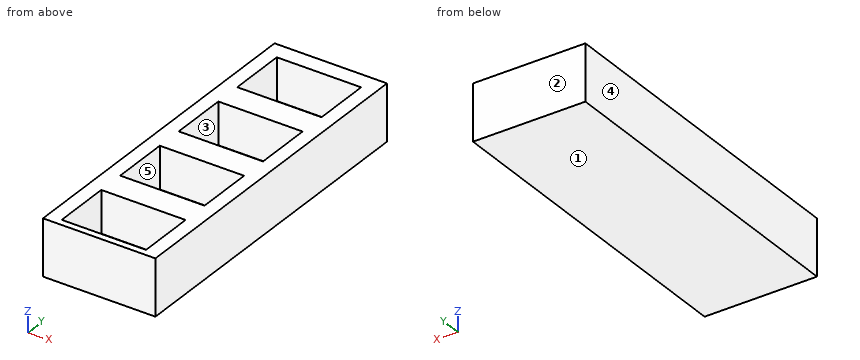
from build123d import *

# Parameters (mm, degrees)
F1_DEPTH = 25.4
F2_DEPTH = 6.35


with BuildPart() as f1:
    # F0 (on Top) → F1 (new body)
    with BuildSketch(Plane.XY):
        Polygon((25.4, -76.2), (25.4, 76.2), (0, 76.2), (-25.4, 76.2), (-25.4, -76.2), align=None)
        Polygon((-19.05, -47.105642), (0, -47.105642), (19.05, -47.105642), (19.05, -73.140642), (-19.05, -73.140642), align=None, mode=Mode.SUBTRACT)
        Polygon((-19.05, -8.599242), (0, -8.599242), (19.05, -8.599242), (19.05, -34.634242), (0, -34.634242), (-19.05, -34.634242), align=None, mode=Mode.SUBTRACT)
        Polygon((-19.05, 29.907158), (0, 29.907158), (19.05, 29.907158), (19.05, 3.872158), (0, 3.872158), (-19.05, 3.872158), align=None, mode=Mode.SUBTRACT)
        Polygon((-19.05, 68.410887), (19.05, 68.410887), (19.05, 42.375887), (0, 42.375887), (-19.05, 42.375887), align=None, mode=Mode.SUBTRACT)
    extrude(amount=F1_DEPTH)

    # F0 (on Top) → F2 (join)
    with BuildSketch(Plane.XY):
        Polygon((19.05, 42.375887), (19.05, 68.410887), (-19.05, 68.410887), (-19.05, 42.375887), (0, 42.375887), align=None)
        Polygon((19.05, 29.907158), (0, 29.907158), (0, 29.675887), (0, 16.889658), (0, 3.872158), (19.05, 3.872158), align=None)
        Polygon((0, 29.675887), (0, 29.907158), (-19.05, 29.907158), (-19.05, 3.872158), (0, 3.872158), (0, 16.889658), align=None)
        Polygon((0, -21.616742), (0, -8.599242), (-19.05, -8.599242), (-19.05, -34.634242), (0, -34.634242), align=None)
        Polygon((19.05, -8.599242), (0, -8.599242), (0, -21.616742), (0, -34.634242), (19.05, -34.634242), align=None)
        Polygon((19.05, -47.105642), (0, -47.105642), (-19.05, -47.105642), (-19.05, -73.140642), (19.05, -73.140642), align=None)
    extrude(amount=F2_DEPTH)


solid = f1.part
Verification items for the finished model (mm, model axes). Face numbers are marked on the shaded views. A direction names the side the tool comes from. Give positions to 0.01 mm unless a question says otherwise; leave off trailing zeros. Loops run counter-clockwise (first coordinate to the right, second up) from the corner with the lowest first, then second, coordinate; pieces in that order, holes last.
1) Sectioned sample at C-C, the plane y = -12. Enter the section's corners in (x, z), then the cut area to 3 significant figures.
2) Sectioned sample at B-B, the plane x = -15.5. Enter the section's corners in (y, z), then the cut area to 3 significant figures.
3) Depth check by flat-ended pin: pin 1 Ø10 at (x, y) = (4, -25.5) entering from -Z; pin 2 Ø3 at (x, y) = (9, 14.5) entering from +Z. Enter the tip coordinate at first touch or a pass-through.
4) Set-up check for the marked faces 4 and 5: record each of +Z, -Z, +X, -X, +Y, -Y from which the full face is reachable in a straight line by a thin tool's end or side.
5) Thickness scan on line 1 along Y through (x, z) = (17, 6.5); line 2 along X through (y, z) = (-26, 17); line 3 along Z through (x, y) = (-14.5, -18). Record the ranges inside material, lowest first.
6) Draft check along Y on the marked faces 1, 2 and 3. Enter one of: pulls with the +Y half, pulls with the -Y half, needs draft (parallel to the pull), parting line crosses it, or undercut.
7) Sectioned sample at A-A, the plane z = 20. Enter the section's corners in (x, y), then the cut area to 3 significant figures.
Answers:
1. outline: (-25.4, 0) - (25.4, 0) - (25.4, 25.4) - (19.05, 25.4) - (19.05, 6.35) - (-19.05, 6.35) - (-19.05, 25.4) - (-25.4, 25.4) - close
1. area: 565 mm2
2. outline: (-76.2, 0) - (76.2, 0) - (76.2, 25.4) - (68.41, 25.4) - (68.41, 6.35) - (42.38, 6.35) - (42.38, 25.4) - (29.91, 25.4) - (29.91, 6.35) - (3.87, 6.35) - (3.87, 25.4) - (-8.6, 25.4) - (-8.6, 6.35) - (-34.63, 6.35) - (-34.63, 25.4) - (-47.11, 25.4) - (-47.11, 6.35) - (-73.14, 6.35) - (-73.14, 25.4) - (-76.2, 25.4) - close
2. area: 1,890 mm2
3. pin 1: stops at z = 0
3. pin 2: stops at z = 6.35
4. face 4: +Z, -Z, -X, +Y, -Y
4. face 5: +Z
5. line 1: y = -76.2 to -73.14, -47.11 to -34.63, -8.6 to 3.87, 29.91 to 42.38, 68.41 to 76.2
5. line 2: x = -25.4 to -19.05, 19.05 to 25.4
5. line 3: z = 0 to 6.35
6. face 1: needs draft
6. face 2: pulls with the +Y half
6. face 3: undercut
7. outline: (-25.4, -76.2) - (25.4, -76.2) - (25.4, 76.2) - (-25.4, 76.2) - close; hole (-19.05, -73.14) - (19.05, -73.14) - (19.05, -47.11) - (-19.05, -47.11) - close; hole (-19.05, -34.63) - (19.05, -34.63) - (19.05, -8.6) - (-19.05, -8.6) - close; hole (-19.05, 3.87) - (19.05, 3.87) - (19.05, 29.91) - (-19.05, 29.91) - close; hole (-19.05, 42.38) - (19.05, 42.38) - (19.05, 68.41) - (-19.05, 68.41) - close
7. area: 3,770 mm2
